```python
from build123d import *

# Parameters (mm, degrees)
SKETCH1_W           = 56
SKETCH1_H           = 30
SKETCH1_W_2         = 42
SKETCH1_H_2         = 22
BOSS_EXTRUDE1_DEPTH = 25.4
BOSS_EXTRUDE2_DEPTH = 56
BOSS_EXTRUDE3_REACH = 67.092
BOSS_EXTRUDE4_DEPTH = 25.4


with BuildPart() as part:
    # Sketch1 → Boss-Extrude1 (new body)
    with BuildSketch(Plane(origin=(0, 0, 0), x_dir=(1, 0, 0), z_dir=(0, 1, 0))):
        Rectangle(SKETCH1_W, SKETCH1_H)
        Rectangle(SKETCH1_W_2, SKETCH1_H_2, mode=Mode.SUBTRACT)
    extrude(amount=BOSS_EXTRUDE1_DEPTH)

    # Sketch2 → Boss-Extrude2 (add)
    with BuildSketch(Plane(origin=(28, 0, 0), x_dir=(0, 0, -1), z_dir=(1, 0, 0))):
        with BuildLine():
            Line((18.175, 22.225), (15, 22.225))
            Line((15, 22.225), (15, 15.875))
            Line((15, 15.875), (18.175, 15.875))
            ThreePointArc((18.175, 15.875), (21.35, 19.05), (18.175, 22.225))
        make_face()
    extrude(amount=-BOSS_EXTRUDE2_DEPTH)

    # Boss-Extrude3: up to this face of the body (flat: up to its plane)
    boss_extrude3_end = Plane(part.part.faces().sort_by_distance((-28, 12.986434698, -0.806465427))[0])
    # Sketch3 → Boss-Extrude3 (add, up to the picked face)
    with BuildSketch(Plane(origin=(28, 0, 0), x_dir=(0, 0, -1), z_dir=(1, 0, 0)), mode=Mode.PRIVATE) as boss_extrude3_sk1:
        with BuildLine():
            Line((15, 25.4), (20.976470588, 36.605882353))
            ThreePointArc((20.976470588, 36.605882353), (19.669117647, 40.901470588), (15.373529412, 39.594117647))
            Line((15.373529412, 39.594117647), (7.803333333, 25.4))
            Line((7.803333333, 25.4), (15, 25.4))
        make_face()
    boss_extrude3_tool1 = split(extrude(boss_extrude3_sk1.sketch, amount=-BOSS_EXTRUDE3_REACH, mode=Mode.PRIVATE), bisect_by=boss_extrude3_end, keep=Keep.BOTH, mode=Mode.PRIVATE)
    add(boss_extrude3_tool1.solids().sort_by(Axis((28, 32.888225, -15.275113), (-1, 0, 0)))[0])

    # Sketch4 → Boss-Extrude4 (add)
    with BuildSketch(Plane.XZ):
        with BuildLine():
            Line((-6.35, 21.35), (-6.35, 15))
            Line((-6.35, 15), (6.35, 15))
            Line((6.35, 15), (6.35, 21.35))
            ThreePointArc((6.35, 21.35), (0, 27.7), (-6.35, 21.35))
        make_face()
    extrude(amount=-BOSS_EXTRUDE4_DEPTH)


solid = part.part
```
For this review, take the finished solid that the model builds, in its own axes (mm). A direction names the side the tool comes from. Give positions to 0.01 mm unless a question says otherwise; leave off trailing zeros. Order: outer loops, then holes, each group sorted by start corner. A loop starts at its lowest first (then second) coordinate and runs counter-clockwise, first axis right, second up.
1) For faces 5 (the face through (0, 13, 11)), 6 (the face through (1.9, 25.4, 11.2)), 7 (the face through (0, 13, -11)), 8 (the face through (0.392, 30.925, -17.946)), list the 3-axis set-ups (+Z, -Z, +X, -X, +Y, -Y) from which the entire face can be reached by the end or side of a thin tool; tool diameter is ignored.
2) Insertion check: pin 1 (1 mm diameter, centred on x = 4, z = -16, fed in from +Y); pin 2 (8 mm diameter, centred on x = -6.5, y = 8, fed in from -Z); pin 3 (3 mm diameter, centred on y = 17.5, z = 17.5, fed in from +X). Each pin has a flat end and moves straight along its axis. Give the tip position at first contact, or say it passes through.
3) Wall thickness on line 1 (Z direction, x = -20, y = 7.5); line 2 (X direction, y = 19.5, z = -8); line 3 (Z direction, x = 23.5, y = 10): over which ranges is each line inside the solid? List them lowest first.
4) Take a section at C-C (y = 19.05). Give the boundary of the cut face in (x, z), then the cut area to 3 significant figures.
5) Take a section at B-B (z = 10). Give the boundary of the cut face in (x, y), then the cut area to 3 significant figures.
6) Take a section at D-D (x = 24.5). Give the boundary of the cut face in (y, z) (3 decimals).
7) Take a section at A-A (x = 0). Give the boundary of the cut face in (y, z) (3 decimals).
8) The part is to be moulded in two halves that separate along Z. For faces 1 (the face through (-6.35, 13, 18)), 2 (the face through (0, 25.4, -9)), 3 (the face through (-21, 13, 0)), 4 (the face through (0.39, 40.87, -19.73)), say which applies: released by +Z, released by -Z, zero draft, split by the parting line, or undercut.
Derived:
1. face 5: +Y, -Y
1. face 6: +Z, +X, -X, +Y
1. face 7: -Y
1. face 8: -Z, +X, -X
2. pin 1: stops at y = 40.8
2. pin 2: stops at z = -15
2. pin 3: stops at x = 6.35
3. line 1: z = -15 to -11, 11 to 15
3. line 2: x = -28 to -21, 21 to 28
3. line 3: z = -15 to 15
4. outline: (-28, -21.35) - (28, -21.35) - (28, 15) - (6.35, 15) - (6.35, 21.35) arc R6.35 ccw to (-6.35, 21.35) - (-6.35, 15) - (-28, 15) - close; hole (-21, -11) - (21, -11) - (21, 11) - (-21, 11) - close
4. area: 1,260 mm2
5. outline: (-28, 0) - (-21, 0) - (-21, 25.4) - (-28, 25.4) - close; (21, 0) - (28, 0) - (28, 25.4) - (21, 25.4) - close
5. area: 356 mm2
6. outline: (0, -15) - (15.875, -15) - (15.875, -18.175) arc R3.175 ccw to (22.225, -18.175) - (22.225, -15) - (25.4, -15) - (36.606, -20.976) arc R3.175 ccw to (39.594, -15.374) - (25.4, -7.803) - (25.4, 15) - (0, 15) - close
7. outline: (0, -15) - (15.875, -15) - (15.875, -18.175) arc R3.175 ccw to (22.225, -18.175) - (22.225, -15) - (25.4, -15) - (36.606, -20.976) arc R3.175 ccw to (39.594, -15.374) - (25.4, -7.803) - (25.4, -11) - (0, -11) - close; (0, 11) - (25.4, 11) - (25.4, 27.7) - (0, 27.7) - close
8. face 1: zero draft
8. face 2: undercut
8. face 3: undercut
8. face 4: split by the parting line
